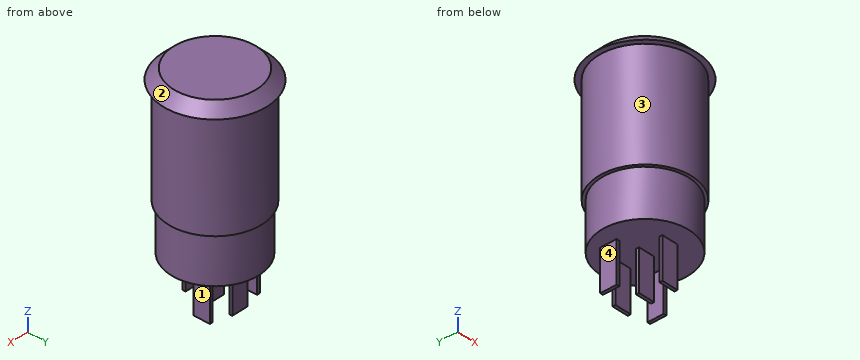
```python
from build123d import *

# Parameters (mm, degrees)
SKETCH_1_R          = 8.9
EXTRUDE_1_DEPTH     = 1.8
EXTRUDE_1_TAPER     = 45
SKETCH_2_R          = 8
EXTRUDE_2_DEPTH     = 26.5
SKETCH_3_W          = 2.8
SKETCH_3_H          = 0.5
SKETCH_3_W_2        = 0.5
SKETCH_3_H_2        = 2.8
EXTRUDE_1_2_DEPTH   = 7
SKETCH_4_R          = 8
SKETCH_4_R_2        = 7.5
CUT_EXTRUDE_1_DEPTH = 8


with BuildPart() as part:
    # 草图1 → Extrude 1 (new body)
    with BuildSketch(Plane.XY):
        Circle(SKETCH_1_R)
    extrude(amount=EXTRUDE_1_DEPTH, taper=EXTRUDE_1_TAPER)

    # 草图2 → 凸台-拉伸2 (add)
    with BuildSketch(Plane(origin=(0, 0, 0), x_dir=(-1, 0, 0), z_dir=(0, 0, -1))):
        Circle(SKETCH_2_R)
    extrude(amount=EXTRUDE_2_DEPTH)

    # 草图3 → Extrude 1 2 (add)
    with BuildSketch(Plane(origin=(0, 0, -26.5), x_dir=(-1, 0, 0), z_dir=(0, 0, -1))):
        Rectangle(SKETCH_3_W, SKETCH_3_H)
        with Locations((0, 4)):
            Rectangle(SKETCH_3_W, SKETCH_3_H)
        with Locations((0, -4)):
            Rectangle(SKETCH_3_W, SKETCH_3_H)
        with Locations((-4.4, 2)):
            Rectangle(SKETCH_3_W_2, SKETCH_3_H_2)
        with Locations((4.4, 2)):
            Rectangle(SKETCH_3_W_2, SKETCH_3_H_2)
    extrude(amount=EXTRUDE_1_2_DEPTH)

    # 草图4 → 切除-拉伸-薄壁1 (cut)
    with BuildSketch(Plane(origin=(0, 0, -26.5), x_dir=(-1, 0, 0), z_dir=(0, 0, -1))):
        Circle(SKETCH_4_R)
        Circle(SKETCH_4_R_2, mode=Mode.SUBTRACT)
    extrude(amount=-CUT_EXTRUDE_1_DEPTH, mode=Mode.SUBTRACT)


solid = part.part
```
Check sheet for the modelled part. Datum: model origin and axes. Units: mm. Face numbers are marked on the shaded views. A direction names the side the tool comes from. Round coordinates to 2 decimals unless told otherwise and drop trailing zeros. Order: outer loops, then holes, each group sorted by start corner. A loop starts at its lowest first (then second) coordinate and runs counter-clockwise, first axis right, second up. Notation, with made-up numbers: (-26, 51) - (-9, 51) arc R5 ccw to (-9, 57) - close; hole circle Ø11 at (59.25, -30). An arc over 180 degrees is marked (long way). Write item = value, one per line.
Q1. Thickness scan on line 1 along X through (y, z) = (1, -31); line 2 along Z through (x, y) = (-2.75, 1); line 3 along Y through (x, z) = (5.75, -9). Record the ranges inside material, lowest first.
Computed:
line_1 = -4.65 to -4.15, 4.15 to 4.65
line_2 = -26.5 to 1.8
line_3 = -5.56 to 5.56
Q2. Section check A-A (x = 0). Record the boundary of the cut face in (y, z), and give its area (3 significant figures).
Computed:
outline = (-8.9, 0) - (-8, 0) - (-8, -18.5) - (-7.5, -18.5) - (-7.5, -26.5) - (-4.25, -26.5) - (-4.25, -33.5) - (-3.75, -33.5) - (-3.75, -26.5) - (-0.25, -26.5) - (-0.25, -33.5) - (0.25, -33.5) - (0.25, -26.5) - (3.75, -26.5) - (3.75, -33.5) - (4.25, -33.5) - (4.25, -26.5) - (7.5, -26.5) - (7.5, -18.5) - (8, -18.5) - (8, 0) - (8.9, 0) - (7.1, 1.8) - (-7.1, 1.8) - close
area = 455 mm^2
Q3. Section check B-B (z = -21). Record the boundary of the cut face in (x, y), and give its area (3 significant figures).
Computed:
outline = circle Ø15 at (0, 0)
area = 177 mm^2
Q4. Go/stop test with flat-tipped pins: pin 1 (10 mm diameter, centred on y = -1.5, z = -23, fed in from +X); pin 2 (4 mm diameter, centred on x = -6.5, z = -13.5, fed in from +Y); pin 3 (2 mm diameter, centred on x = 4.5, y = -4.5, fed in from -Z). Record where each tip stops, or that it passes through.
Computed:
pin_1 = 8
pin_2 = 6.61
pin_3 = -26.5
Q5. Section check C-C (z = -15). Record the boundary of the cut face in (x, y).
Computed:
outline = circle Ø16 at (0, 0)
Q6. Tool access check on the marked faces 1, 2, 3 and 4. Record the directions out of +Z, -Z, +X, -X, +Y, -Y that give a thin tool (end or side, any length) a straight path to the whole face; none if there is none.
Computed:
face_1 = -Z, +X, +Y, -Y
face_2 = +Z
face_3 = -Z
face_4 = -Z, -X, +Y, -Y
